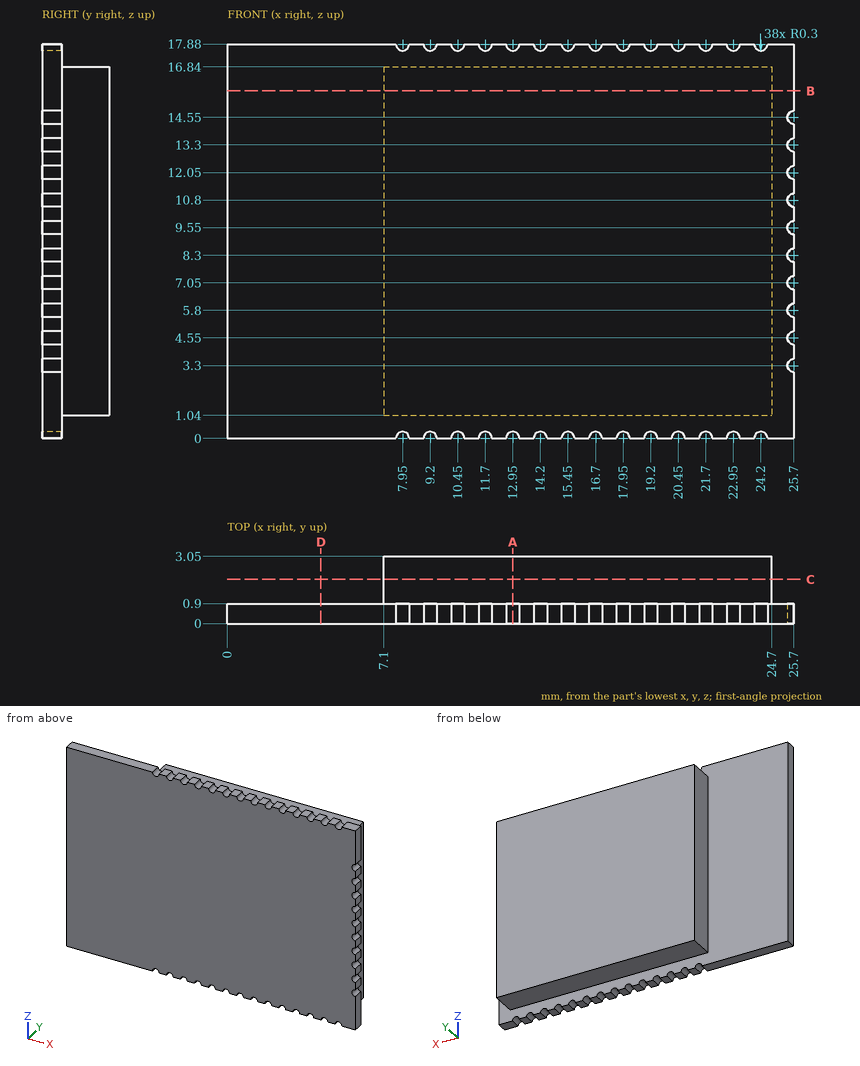
Check sheet for the drawn part. Datum: minimum x, y, z corner. Units: mm. Round coordinates to 2 decimals unless told otherwise and drop trailing zeros. Write each loop counter-clockwise with the first axis right and the second up, starting at its lowest first coordinate (ties: lowest second). Pieces come first, ordered by that corner, then holes. Notation, with made-up numbers: (20, 88) - (38, 88) arc R35 cw to (38, 121) - close; hole circle Ø11 at (-37.5, 42.25). An arc over 180 degrees is marked (long way). Write each question's results on one line, items separated by ' | '.
(1) Sectioned sample at B-B, the plane z = 15.75. Enter the section's corners in (x, y), plus the area to 3 significant figures.
Computed:
outline: (0, 0) - (25.7, 0) - (25.7, 0.9) - (24.7, 0.9) - (24.7, 3.05) - (7.1, 3.05) - (7.1, 0.9) - (0, 0.9) - close | area: 61.0 mm^2
(2) Thickness scan on probe 1 along Y at (x, z) = (4.75, 17); probe 2 along X at (y, z) = (1.7, 3.75); probe 3 along X at (y, z) = (0.5, 3.25). Record the ranges inside material, lowest first. Write a range as from..to.
Computed:
probe 1: y = 0..0.9 | probe 2: x = 7.1..24.7 | probe 3: x = 0..25.4
(3) Sectioned sample at C-C, the plane y = 2. Enter the section's corners in (x, z), plus the area to 3 significant figures.
Computed:
outline: (7.1, 1.04) - (24.7, 1.04) - (24.7, 16.84) - (7.1, 16.84) - close | area: 278 mm^2
(4) Depth check by flat-ended pin: pin 1 Ø5 at (x, z) = (7, 10.5) entering from +Y; pin 2 Ø1.7 at (x, y) = (19, 2) entering from -Z; pin 3 Ø0.6 at (y, z) = (2, 8.5) entering from -X; pin 4 Ø1.7 at (y, z) = (2, 11.5) entering from +X. Enter the tip coordinate at first touch or a pass-through.
Computed:
pin 1: stops at y = 3.05 | pin 2: stops at z = 1.04 | pin 3: stops at x = 7.1 | pin 4: stops at x = 24.7
(5) Sectioned sample at A-A, the plane x = 12.95. Enter the section's corners in (y, z), plus the area to 3 significant figures.
Computed:
outline: (0, 0.3) - (0.9, 0.3) - (0.9, 1.04) - (3.05, 1.04) - (3.05, 16.84) - (0.9, 16.84) - (0.9, 17.58) - (0, 17.58) - close | area: 49.5 mm^2
(6) Sectioned sample at D-D, the plane x = 4.25. Enter the section's corners in (y, z), plus the area to 3 significant figures.
Computed:
outline: (0, 0) - (0.9, 0) - (0.9, 17.88) - (0, 17.88) - close | area: 16.1 mm^2
